For this review, use the dimensioned drawing (mm, ordinates from the lowest corner) and the shaded views. A direction names the side the tool comes from. Round coordinates to 2 decimals unless told otherwise and drop trailing zeros. Write each loop counter-clockwise with the first axis right and the second up, starting at its lowest first coordinate (ties: lowest second). Pieces come first, ordered by that corner, then holes.
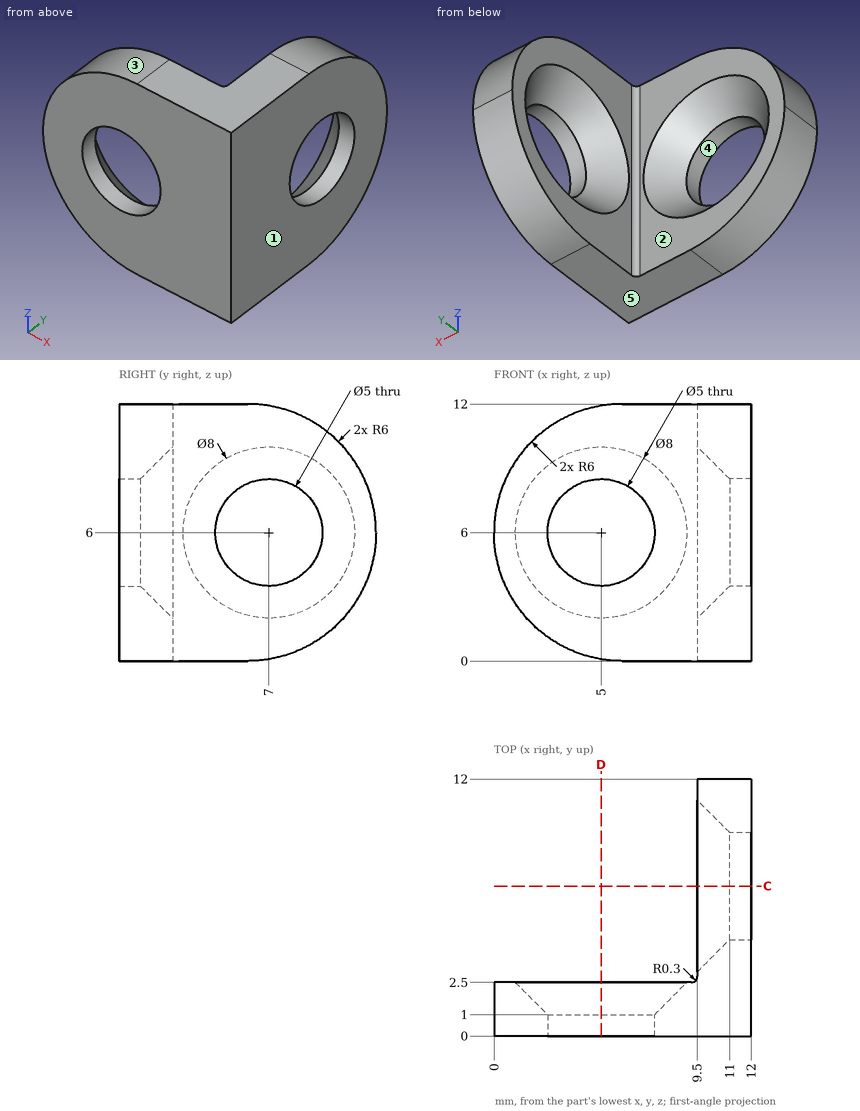
(1) We need section D-D, the plane x = 5. Give the boundary of the cut face in (y, z), and give its area (3 significant figures).
Geometry check:
outline: (0, 0.08) - (2.5, 0.08) - (2.5, 2) - (1, 3.5) - (0, 3.5) - close; (0, 8.5) - (1, 8.5) - (2.5, 10) - (2.5, 11.92) - (0, 11.92) - close
area: 14.8 mm2
(2) For line 1 along Y through (x, z) = (0.5, 5.75); line 2 along Z through (x, y) = (9.75, 8); line 3 along Z through (x, y) = (11.75, 7), list the stretches that pass through material, from the lowest coordinate up.
Geometry check:
line 1: y = 0 to 2.5
line 2: z = 0.34 to 2.39, 9.61 to 11.66
line 3: z = 0.08 to 3.5, 8.5 to 11.92
(3) For pin 1 Ø2 at (x, z) = (2, 4.5) entering from +Y; pin 2 Ø3 at (x, y) = (7, 6) entering from -Z; pin 3 Ø3 at (y, z) = (5.5, 5.5) entering from -X, all flat-tipped, find the tip position at first contact; note any pin that passes through.
Geometry check:
pin 1: stops at y = 2.5
pin 2: passes through
pin 3: stops at x = 10.42
(4) Mouldability with a two-part tool opening along X and no side actions: class the marked faces 3, 4 and 5 as pulls with the +X half, pulls with the -X half, needs draft (parallel to the pull), parting line crosses it, or undercut.
Geometry check:
face 3: pulls with the -X half
face 4: undercut
face 5: needs draft
(5) For the marked faces 1 and 2, list the 3-axis set-ups (+Z, -Z, +X, -X, +Y, -Y) from which the entire face can be reached by the end or side of a thin tool; tool diameter is ignored.
Geometry check:
face 1: +Z, -Z, +X, +Y, -Y
face 2: +Z, -Z, -X, +Y
(6) We need section C-C, the plane y = 7. Give the boundary of the cut face in (x, z), and give its area (3 significant figures).
Geometry check:
outline: (9.5, 0.08) - (12, 0.08) - (12, 3.5) - (11, 3.5) - (9.5, 2) - close; (9.5, 10) - (11, 8.5) - (12, 8.5) - (12, 11.92) - (9.5, 11.92) - close
area: 14.8 mm2
